```python
from build123d import *

# Parameters (mm, degrees)
F0_W     = 86.981553
F0_H     = 39.354872
F1_DEPTH = 25
F2_T     = -2.5
F3_R     = 7.757287
F4_DEPTH = 25
F6_DEPTH = 25


with BuildPart() as f1:
    # F0 (on Front) → F1 (new body)
    with BuildSketch(Plane.XZ):
        with Locations((-93.148147, -0.701256)):
            Rectangle(F0_W, F0_H)
    extrude(amount=F1_DEPTH)

    # F2
    f2_openings = [f1.faces().sort_by_distance(p)[0] for p in [
        (-93.148148, -25, -0.701256),
    ]]
    offset(amount=F2_T, openings=f2_openings)

    # F3 (on face) → F4 (cut)
    with BuildSketch(Plane.XZ.offset(2.5)):
        with Locations((-98.527715, -0.701256)):
            Circle(F3_R)
    extrude(amount=-F4_DEPTH, mode=Mode.SUBTRACT)

    # F5 (on face) → F6 (cut)
    with BuildSketch(Plane.XZ.offset(2.5)):
        Polygon((-119.016969, -5.981139), (-114.744506, -2.821497), (-115.344604, 2.458386), (-120.217166, 4.578626), (-124.489629, 1.418985), (-123.889531, -3.860898), align=None)
        Polygon((-65.501607, -8.603557), (-61.395115, -5.566656), (-61.209103, -0.462595), (-65.083642, 2.865165), (-70.101126, 1.910753), (-72.483286, -2.60714), (-70.436308, -7.286448), align=None)
    extrude(amount=-F6_DEPTH, mode=Mode.SUBTRACT)


solid = f1.part
```
Geometry: final body of the model. Coordinates: model frame, mm. A direction names the side the tool comes from. Round coordinates to 2 decimals unless told otherwise and drop trailing zeros. Write each loop counter-clockwise with the first axis right and the second up, starting at its lowest first coordinate (ties: lowest second). Pieces come first, ordered by that corner, then holes. Notation, with made-up numbers: (14.25, 23) -> (71.25, 23) arc R16 cw to (71.25, 48) -> close; hole circle Ø2 at (-16, 5). An arc over 180 degrees is marked (long way). Use CSV: the item, a comma, the result in double quotes. Start each with the question number.
Q1. Section C-C (z = -10.5). Return loops of the section in (x, y), plus the area to 3 significant figures.
Q2. Section D-D (x = -95.5). Return loops of the section in (y, z).
Q3. Section B-B (x = -75.5). Return loops of the section in (y, z).
Q4. Pull-direction query (X, two-part tool) for faces 1 (the face through (-136.639, -12, -1)), 2 (the face through (-96.6, -25, -18.1)), 3 (the face through (-122.323, -1.268, 3.021)); classes: pulls with the +X half, pulls with the -X half, needs draft (parallel to the pull), parting line crosses it, or undercut.
Q5. Section A-A (y = -9). Return loops of the section in (x, z).
Q6. Reachability of faces 4 (the face through (-124.194, -1.268, -1.184)), 5 (the face through (-49.657, -12, -1)), 6 (the face through (-52.157, -14, -1)) from +Z, -Z, +X, -X, +Y, -Y: full face, straight path, thin tool, end or side. Return the list, or none.
Q7. Line query: L1, parallel to X at y = -11.5, z = 1; L2, parallel to Z at x = -63.5, y = -20; L3, parallel to Y at x = -54.5, z = 13.5. Output: solid intervals per line, ascending.
Q8. First-contact query: pin 1 Ø14 at (x, z) = (-98.53, -0.7) entering from +Y; pin 2 Ø5 at (x, z) = (-108, -12) entering from -Y; pin 3 Ø3 at (x, z) = (-65.5, 6) entering from +Y. Flat tips, straight axial feed; report the tip coordinate or a pass-through.
Result sheet:
1,outline,"(-136.64, -25) -> (-134.14, -25) -> (-134.14, -2.5) -> (-52.16, -2.5) -> (-52.16, -25) -> (-49.66, -25) -> (-49.66, 0) -> (-136.64, 0) -> close"
1,area,"330 mm²"
2,outline,"(-25, -20.38) -> (0, -20.38) -> (0, -7.84) -> (-2.5, -7.84) -> (-2.5, -17.88) -> (-25, -17.88) -> close; (-25, 16.48) -> (-2.5, 16.48) -> (-2.5, 6.44) -> (0, 6.44) -> (0, 18.98) -> (-25, 18.98) -> close"
3,outline,"(-25, -20.38) -> (0, -20.38) -> (0, 18.98) -> (-25, 18.98) -> (-25, 16.48) -> (-2.5, 16.48) -> (-2.5, -17.88) -> (-25, -17.88) -> close"
4,face 1,"pulls with the -X half"
4,face 2,"needs draft"
4,face 3,"undercut"
5,outline,"(-136.64, -20.38) -> (-49.66, -20.38) -> (-49.66, 18.98) -> (-136.64, 18.98) -> close; hole (-134.14, -17.88) -> (-52.16, -17.88) -> (-52.16, 16.48) -> (-134.14, 16.48) -> close"
6,face 4,"+Y, -Y"
6,face 5,"+Z, -Z, +X, +Y, -Y"
6,face 6,"-Y"
7,L1,"-136.64 to -134.14, -52.16 to -49.66"
7,L2,"-20.38 to -17.88, 16.48 to 18.98"
7,L3,"-2.5 to 0"
8,pin 1,"through"
8,pin 2,"y = -2.5"
8,pin 3,"y = 0"
